Autodesk Inventor part; units mm, degrees
ref_plane "YZ Plane" through (0, 0, 0) normal (1, 0, 0) x (0, 1, 0)
ref_plane "XZ Plane" through (0, 0, 0) normal (0, 1, 0) x (-1, 0, 0)
ref_plane "XY Plane" through (0, 0, 0) normal (0, 0, 1) x (1, 0, 0)
sketch "Sketch1" plane through (0, 0, 0) normal (0, 0, 1) x (1, 0, 0)
  circle A0 centre (0, 0) radius 4
  circle A1 centre (0, 0) radius 11
  dimension "d0" = 8
  dimension "d1" = 22
extrude "Extrusion1" add sketch "Sketch1" along normal blind 3.6
sketch "Sketch2" plane through (0, 0, 3.6) normal (0, 0, 1) x (1, 0, 0)
  circle A0 centre (0, 0) radius 4
  circle A1 centre (0, 0) radius 11
  circle A2 centre (0, 0) radius 5.15
  dimension "d4" = 10.3
extrude "Extrusion2" add sketch "Sketch2" along normal blind 10 contours A2
sketch "Sketch3" plane through (0, 0, 3.6) normal (0, 0, 1) x (1, 0, 0)
  circle A0 centre (0, 0) radius 5.15
  circle A1 centre (0, 0) radius 11
  circle A2 centre (0, 8) radius 1.625
  dimension "d7" = 3.25
  dimension "d8" = 8
extrude "Extrusion3" cut sketch "Sketch3" against normal blind 10 contours A2
pattern_circular "Circular Pattern1" count 4 over 360 about axis through (0, 0, 3.6) along (0, 0, 1) of "Extrusion3"
properties part number "00_spindel_slide"
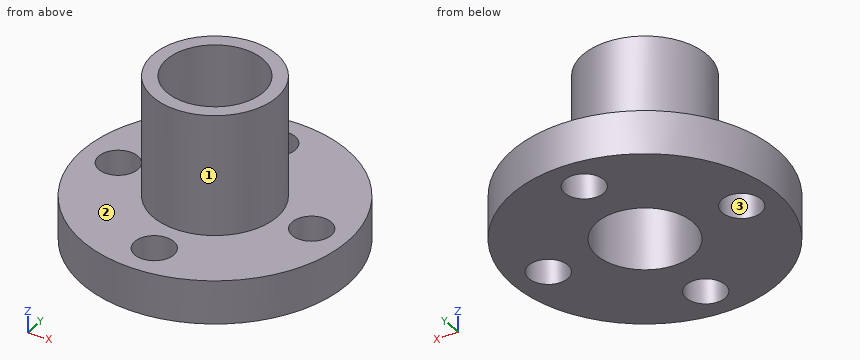
The listing builds one solid part. Answer for the finished solid, in the listing's coordinates (mm). Face numbers are marked on the shaded views. Coordinates: 2 decimals unless noted, no trailing zeros. Loops run counter-clockwise (first coordinate to the right, second up) from the corner with the lowest first, then second, coordinate; pieces in that order, holes last. Notation, with made-up numbers: (84, 7.25) -> (134, 7.25) arc R37 ccw to (134, 43.25) -> close; hole circle Ø9 at (27.5, 11.5). An arc over 180 degrees is marked (long way). Answer in a Markdown table with one row per item. Add a question column.
1. The part is cut by section B-B, the plane x = 8. Write down the section's boundary in (y, z) (3 decimals), then the cut area to 3 significant figures.
2. Determine the mould class of the marked faces 1, 2 and 3 for opening direction Y: +Y half, -Y half, draft (parallel to the pull), parting line (faces both ways), or undercut.
3. The part is cut by section C-C, the plane z = 1.75. Write down the section's boundary in (x, y) (3 decimals).
4. The part is cut by section A-A, the plane y = 0. Write down the section's boundary in (x, z) (3 decimals).
5. Consider line 1 (Y direction, x = 0, z = 9); line 2 (Z direction, x = -6, y = 5.5); line 3 (Y direction, x = -8, z = 1.6) (3 decimals). Determine where each line is inside the solid, lowest interval first. Write a range as [from, to].
6. Flat-ended cylindrical pins translate along their axes: P1, Ø1, axis at x = -1, y = -5, coming from the -Z side; P2, Ø3, axis at x = 0, y = 8, coming from the +Z side; P3, Ø5, axis at x = 8, y = 0, coming from the +Z side; P4, Ø1.5, axis at y = -0.5, z = 8.5, coming from the +X side. Find the tip coordinate at first contact, or state that the pin passes through.
Answer below:
| question | item | result |
|---|---|---|
| 1 | outline | (-7.55, 0) -> (-1.625, 0) -> (-1.625, 3.6) -> (-7.55, 3.6) -> close; (1.625, 0) -> (7.55, 0) -> (7.55, 3.6) -> (1.625, 3.6) -> close |
| 1 | area | 42.7 mm2 |
| 2 | face 1 | parting line |
| 2 | face 2 | draft |
| 2 | face 3 | undercut |
| 3 | outline | circle Ø22 at (0, 0); hole circle Ø3.25 at (-8, 0); hole circle Ø8 at (0, 0); hole circle Ø3.25 at (0, -8); hole circle Ø3.25 at (0, 8); hole circle Ø3.25 at (8, 0) |
| 4 | outline | (-11, 0) -> (-9.625, 0) -> (-9.625, 3.6) -> (-11, 3.6) -> close; (-6.375, 0) -> (-4, 0) -> (-4, 13.6) -> (-5.15, 13.6) -> (-5.15, 3.6) -> (-6.375, 3.6) -> close; (4, 0) -> (6.375, 0) -> (6.375, 3.6) -> (5.15, 3.6) -> (5.15, 13.6) -> (4, 13.6) -> close; (9.625, 0) -> (11, 0) -> (11, 3.6) -> (9.625, 3.6) -> close |
| 5 | line 1 | [-5.15, -4], [4, 5.15] |
| 5 | line 2 | [0, 3.6] |
| 5 | line 3 | [-7.55, -1.625], [1.625, 7.55] |
| 6 | P1 | z = 0 |
| 6 | P2 | through |
| 6 | P3 | z = 3.6 |
| 6 | P4 | x = 5.15 |
